from build123d import *

# Parameters (mm, degrees)
ESQUISSE1_R        = 1.15
BOSS_EXTRU_1_DEPTH = 6
CONG_1_R           = 5


with BuildPart() as part:
    # Esquisse1 → Boss.-Extru.1 (new body)
    with BuildSketch(Plane.XY):
        with BuildLine():
            Line((-58.352913381, 15), (-54.346688032, 18))
            ThreePointArc((-54.346688032, 18), (0, 57.25), (54.346688032, 18))
            Line((54.346688032, 18), (58.352913381, 15))
            ThreePointArc((58.352913381, 15), (60.25, 0), (58.352913381, -15))
            Line((58.352913381, -15), (54.346688032, -18))
            ThreePointArc((54.346688032, -18), (0, -57.25), (-54.346688032, -18))
            Line((-54.346688032, -18), (-58.352913381, -15))
            ThreePointArc((-58.352913381, -15), (-60.25, 0), (-58.352913381, 15))
        make_face()
        with Locations((0, 53.85)):
            Circle(ESQUISSE1_R, mode=Mode.SUBTRACT)
        with Locations((46.635467994, 26.925)):
            Circle(ESQUISSE1_R, mode=Mode.SUBTRACT)
        with Locations((46.635467994, -26.925)):
            Circle(ESQUISSE1_R, mode=Mode.SUBTRACT)
        with Locations((0, -53.85)):
            Circle(ESQUISSE1_R, mode=Mode.SUBTRACT)
        with Locations((-46.635467994, -26.925)):
            Circle(ESQUISSE1_R, mode=Mode.SUBTRACT)
        with Locations((-46.635467994, 26.925)):
            Circle(ESQUISSE1_R, mode=Mode.SUBTRACT)
    extrude(amount=BOSS_EXTRU_1_DEPTH)

    # Congé1
    cong_1_edges = [part.edges().sort_by_distance(p)[0] for p in [
        (-54.346688032, -18, 3),
        (-58.352913381, -15, 3),
        (-58.352913381, 15, 3),
        (-54.346688032, 18, 3),
        (54.346688032, 18, 3),
        (58.352913381, 15, 3),
        (58.352913381, -15, 3),
        (54.346688032, -18, 3),
    ]]
    fillet(cong_1_edges, radius=CONG_1_R)


solid = part.part
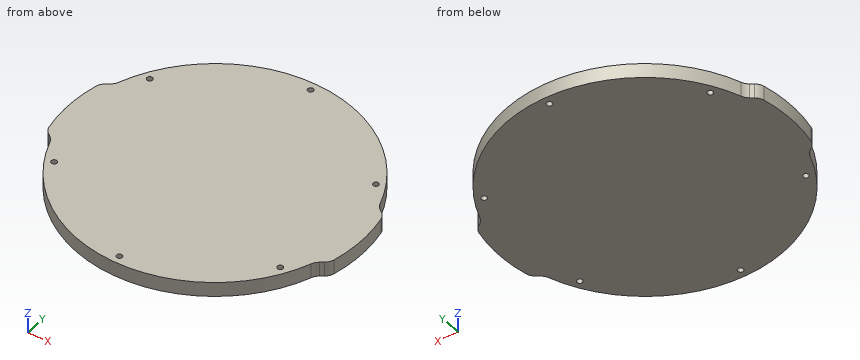
Design review of the part built by this model. Coordinates are the model's own, in mm. Give positions to 0.01 mm unless a question says otherwise; leave off trailing zeros. Write each loop counter-clockwise with the first axis right and the second up, starting at its lowest first coordinate (ties: lowest second). Pieces come first, ordered by that corner, then holes. Notation, with made-up numbers: M -9.75,-26 L -1.75,-26 A14 ccw -1.75,-12 Z; hole C 74.5,50 d10. An arc over 180 degrees is marked long. Return JSON: item names as keys, results as strings. Group by question number.
Item 1: Take a section at B-B (x = 32). Give the boundary of the cut face in (y, z), plus the area to 3 significant figures.
Item 2: Clearance check with flat-ended pins moving along their axes: pin 1 Ø1 at (y, z) = (-42, 1) entering from -X; pin 2 Ø1.5 at (x, z) = (-24, 3) entering from +Y. State where each tip first meets the part, or that it passes through.
Item 3: Take a section at C-C (y = -34). Give the boundary of the cut face in (x, z), plus the area to 3 significant figures.
Item 4: Wall thickness on line 1 along X through (y, z) = (-1, 1.05); line 2 along X through (y, z) = (36, 2.45); line 3 along Y through (x, z) = (-10, 2.05): over which ranges is each line inside the solid? List them lowest first.
Item 5: Take a section at A-A (z = 1.9). Count the separate pieces of the cut face and the enclosed holes in it, plus the area to 3 significant figures.
Return value:
{
 "1": {"outline": "M -47.47,0 L 47.47,0 L 47.47,6 L -47.47,6 Z", "area": "570 mm2"},
 "2": {"pin 1": "stops at x = -39.44", "pin 2": "stops at y = 52.32"},
 "3": {"outline": "M -46.06,0 L 46.06,0 L 46.06,6 L -46.06,6 Z", "area": "553 mm2"},
 "4": {"line 1": "x = -60.24 to 60.24", "line 2": "x = -44.51 to 44.51", "line 3": "y = -56.37 to 56.37"},
 "5": {"separate pieces": "1", "enclosed holes": "6", "area": "10,500 mm2"}
}
